Could you check a few things on this model? Use its own coordinates, in mm. A direction names the side the tool comes from. Coordinates: 2 decimals unless noted, no trailing zeros. Loops run counter-clockwise (first coordinate to the right, second up) from the corner with the lowest first, then second, coordinate; pieces in that order, holes last. Notation, with made-up numbers: (16, 46.5) - (22, 46.5) arc R11 ccw to (22, 64.5) - close; hole circle Ø4 at (23, 50). An arc over 180 degrees is marked (long way). Use CSV: the item, a comma, the result in double quotes.
from build123d import *

# Parameters (mm, degrees)
F0_W     = 61.468017
F0_H     = 61.468017
F0_W_2   = 36.068017
F0_H_2   = 36.068017
F1_DEPTH = 12.7
F2_R     = 2.54
F3_DEPTH = 11.43


with BuildPart() as f1:
    # F0 (on Top) → F1 (new body)
    with BuildSketch(Plane.XY):
        with Locations((7.701496, 11.267003)):
            Rectangle(F0_W, F0_H)
        with Locations((7.701497, 11.267004)):
            Rectangle(F0_W_2, F0_H_2, mode=Mode.SUBTRACT)
    extrude(amount=F1_DEPTH)

    # F2 (on face) → F3 (cut)
    with BuildSketch(Plane.XY.offset(12.7)):
        with Locations((-16.682512, 35.651012)):
            Circle(F2_R)
        with Locations((32.085505, 35.651012)):
            Circle(F2_R)
        with Locations((32.085505, -13.117005)):
            Circle(F2_R)
        with Locations((-16.682512, -13.117005)):
            Circle(F2_R)
    extrude(amount=-F3_DEPTH, mode=Mode.SUBTRACT)


solid = f1.part
(1) Suppose I cut it at C-C (z = 7). Write out the boundary of the cut face in (x, y), plus the area to 3 significant figures.
Computed:
outline,"(-23.03, -19.47) - (38.44, -19.47) - (38.44, 42) - (-23.03, 42) - close; hole circle Ø5.08 at (-16.68, -13.12); hole circle Ø5.08 at (-16.68, 35.65); hole (-10.33, -6.77) - (25.74, -6.77) - (25.74, 29.3) - (-10.33, 29.3) - close; hole circle Ø5.08 at (32.09, -13.12); hole circle Ø5.08 at (32.09, 35.65)"
area,"2,400 mm²"
(2) Will this pin go through, and if not, where does the flat tip stop? pin 1 (2.5 mm diameter, centred on x = 32, y = 35.5, fed in from +Z).
Computed:
pin 1,"stops at z = 1.27"
(3) Please list where these lines run through material, in increasing order: line 1 (Y direction, x = 32, z = 1.5); line 2 (X direction, y = -3, z = 5); line 3 (Y direction, x = 8.5, z = 4.5).
Computed:
line 1,"y = -19.47 to -15.66, -10.58 to 33.11, 38.19 to 42"
line 2,"x = -23.03 to -10.33, 25.74 to 38.44"
line 3,"y = -19.47 to -6.77, 29.3 to 42"
(4) Which directions (+Z, -Z, +X, -X, +Y, -Y) give clear straight access to the entire face, cutting with the end or side of a thin tool? Please do faces 4 (the face through (-17.01, -10.6, 7.07)), 5 (the face through (38.436, 11, 6)), 6 (the face through (7, 29.301, 6)).
Computed:
face 4,"+Z"
face 5,"+Z, -Z, +X, +Y, -Y"
face 6,"+Z, -Z"
(5) Thinking about a two-plate mould opening in Y: for faces 1 (the face through (-13, 12, 0)), 2 (the face through (31.75, -10.6, 7.07)), 3 (the face through (7, 42.001, 6)), which applies, +Y half, -Y half, draft (parallel to the pull), parting line (faces both ways), or undercut?
Computed:
face 1,"draft"
face 2,"undercut"
face 3,"+Y half"
(6) Suppose I cut it at A-A (x = 16). Write out the boundary of the cut face in (y, z), plus the area to 3 significant figures.
Computed:
outline,"(-19.47, 0) - (-6.77, 0) - (-6.77, 12.7) - (-19.47, 12.7) - close; (29.3, 0) - (42, 0) - (42, 12.7) - (29.3, 12.7) - close"
area,"323 mm²"
(7) Suppose I cut it at B-B (y = 20.5). Write out the boundary of the cut face in (x, z).
Computed:
outline,"(-23.03, 0) - (-10.33, 0) - (-10.33, 12.7) - (-23.03, 12.7) - close; (25.74, 0) - (38.44, 0) - (38.44, 12.7) - (25.74, 12.7) - close"
(8) Suppose I cut it at D-D (x = -15.5). Write out the boundary of the cut face in (y, z).
Computed:
outline,"(-19.47, 0) - (42, 0) - (42, 12.7) - (37.9, 12.7) - (37.9, 1.27) - (33.4, 1.27) - (33.4, 12.7) - (-10.87, 12.7) - (-10.87, 1.27) - (-15.36, 1.27) - (-15.36, 12.7) - (-19.47, 12.7) - close"
